Source: CAD feature listing. Evaluate the final solid. Frame: model axes, mm. Coordinates: 2 decimals unless noted, no trailing zeros. Loops run counter-clockwise (first coordinate to the right, second up) from the corner with the lowest first, then second, coordinate; pieces in that order, holes last. Notation, with made-up numbers: (70.5, 8.25) - (111.5, 8.25) arc R20 ccw to (111.5, 24.25) - close; hole circle Ø10 at (-2.75, 2). An arc over 180 degrees is marked (long way). Write item = value, one per line. Start each with the question number.
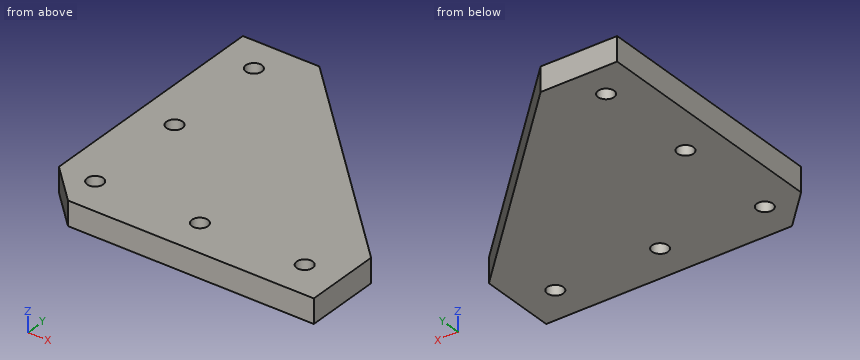
from build123d import *

# Parameters (mm, degrees)
SKETCH1_R           = 2
BOSS_EXTRUDE1_DEPTH = 6
CHAMFER1_SIZE       = 9


with BuildPart() as part:
    # Sketch1 → Boss-Extrude1 (new body)
    with BuildSketch(Plane.XY):
        Polygon((0, 70), (0, 0), (70, 0), (70, 19), (19, 70), align=None)
        with Locations((9, 9)):
            Circle(SKETCH1_R, mode=Mode.SUBTRACT)
        with Locations((35, 9)):
            Circle(SKETCH1_R, mode=Mode.SUBTRACT)
        with Locations((61, 9)):
            Circle(SKETCH1_R, mode=Mode.SUBTRACT)
        with Locations((9, 61.643837586)):
            Circle(SKETCH1_R, mode=Mode.SUBTRACT)
        with Locations((9, 35.321918793)):
            Circle(SKETCH1_R, mode=Mode.SUBTRACT)
    extrude(amount=BOSS_EXTRUDE1_DEPTH)

    # Chamfer1
    chamfer1_edges = [part.edges().sort_by_distance(p)[0] for p in [
        (0, 0, 3),
    ]]
    chamfer(chamfer1_edges, length=CHAMFER1_SIZE)


solid = part.part
Item 1: Cut plane B-B (y = 36.5). Return the cut outline in (x, z).
Item 2: First-contact query: pin 1 (4.5 mm diameter, centred on x = 9, y = 9, fed in from -Z). Flat tip, straight axial feed; report the tip coordinate or a pass-through.
Item 3: Material intervals for L1, parallel to Y at x = 9, z = 2.35; L2, parallel to X at y = 10.5, z = 1.65; L3, parallel to Y at x = 9.5, z = 2.75, sorted ascending. Write a range as [from, to].
Item 4: Cut plane C-C (z = 4.25). Return the cut outline in (x, y), then the cut area to 3 significant figures.
Item 5: Cut plane A-A (x = 35). Return the cut outline in (y, z), then the cut area to 3 significant figures.
Item 6: Cut plane D-D (y = 22). Return the cut outline in (x, z), then the cut area to 3 significant figures.
Responses:
q1.outline = (0, 0) - (7.38, 0) - (7.38, 6) - (0, 6) - close; (10.62, 0) - (52.5, 0) - (52.5, 6) - (10.62, 6) - close
q2.pin_1 = 0
q3.L1 = [0, 7], [11, 33.32], [37.32, 59.64], [63.64, 70]
q3.L2 = [0, 7.68], [10.32, 33.68], [36.32, 59.68], [62.32, 70]
q3.L3 = [0, 7.06], [10.94, 33.39], [37.26, 59.71], [63.58, 70]
q4.outline = (0, 9) - (9, 0) - (70, 0) - (70, 19) - (19, 70) - (0, 70) - close; hole circle Ø4 at (9, 9); hole circle Ø4 at (9, 35.32); hole circle Ø4 at (9, 61.64); hole circle Ø4 at (35, 9); hole circle Ø4 at (61, 9)
q4.area = 3,500 mm2
q5.outline = (0, 0) - (7, 0) - (7, 6) - (0, 6) - close; (11, 0) - (54, 0) - (54, 6) - (11, 6) - close
q5.area = 300 mm2
q6.outline = (0, 0) - (67, 0) - (67, 6) - (0, 6) - close
q6.area = 402 mm2
